CAD build for the part. Positions are in the model's coordinates, mm. A direction names the side the tool comes from. Round coordinates to 2 decimals unless told otherwise and drop trailing zeros. Order: outer loops, then holes, each group sorted by start corner. A loop starts at its lowest first (then second) coordinate and runs counter-clockwise, first axis right, second up. Notation, with made-up numbers: (-3.75, -37.5) -> (24.25, -37.5) arc R31 cw to (24.25, -6.5) -> close; hole circle Ø2 at (82, -5). An arc over 180 degrees is marked (long way). Return JSON: item names as keys, results as strings. Group by question number.
Q1. Cut at B-B (z = -3.75). Write the cut outline in (x, y) (3 decimals), then the cut area to 3 significant figures.
Q2. Cut at C-C (y = 25.4). Write the cut outline in (x, z) (3 decimals).
Q3. Flat gauge pin, fed straight in: pin 1 (4 mm diameter, centred on y = -66.675, z = 3.175, fed in from +X). Where does the tip first touch, or does it go through?
Q4. Cut at A-A (x = 0). Write the cut outline in (y, z) (3 decimals), then the cut area to 3 significant figures.
Q5. Which spindle directions (+Z, -Z, +X, -X, +Y, -Y) get a long thin tool onto all of the face, cutting with end or side? Do faces 5 (the flat face through (-22.225, 1, 0)), 6 (the flat face through (0, 76.2, -10)). Say none if no direction does.
Q6. Mould opens along Y. For faces 1 (the cylindrical face through (-23.835, 28.548, 2.762)), 2 (the flat face through (0, 1, 9.525)), 3 (the flat face through (0, -76.2, -10)), 4 (the cylindrical face through (23.79, 28.548, 2.762)) say: +Y half, -Y half, draft (parallel to the pull), parting line (faces both ways), or undercut.
Q7. Cut at D-D (z = 4.75). Write the cut outline in (x, y) (3 decimals).
Q8. Probe line 1 along X through (y, z) = (-0.5, 3) (3 decimals); line 2 along Z through (x, y) = (5.5, 43.5) (3 decimals). List the from-to ranges inside material, lowest first.
from build123d import *

# Parameters (mm, degrees)
SKETCH1_W           = 50.8
SKETCH1_H           = 25.4
SKETCH1_W_2         = 44.45
SKETCH1_H_2         = 19.05
BOSS_EXTRUDE1_DEPTH = 76.2
SKETCH2_R           = 3.175
CUT_EXTRUDE1_DEPTH  = 93.457395594


with BuildPart() as part:
    # Sketch1 → Boss-Extrude1 (new, symmetric)
    with BuildSketch(Plane(origin=(0, 0, 0), x_dir=(1, 0, 0), z_dir=(0, 1, 0))):
        Rectangle(SKETCH1_W, SKETCH1_H)
        Rectangle(SKETCH1_W_2, SKETCH1_H_2, mode=Mode.SUBTRACT)
    extrude(amount=BOSS_EXTRUDE1_DEPTH, both=True)

    # Sketch2 → Cut-Extrude1 (cut, through all)
    with BuildSketch(Plane.ZY.offset(25.4)):
        with Locations((3.175, -66.675)):
            Circle(SKETCH2_R)
        with Locations((3.175, 25.4)):
            Circle(SKETCH2_R)
    extrude(amount=-CUT_EXTRUDE1_DEPTH, mode=Mode.SUBTRACT)


solid = part.part
Solution:
{
 "1": {"outline": "(-25.4, -76.2) -> (-22.225, -76.2) -> (-22.225, 76.2) -> (-25.4, 76.2) -> close; (22.225, -76.2) -> (25.4, -76.2) -> (25.4, 76.2) -> (22.225, 76.2) -> close", "area": "968 mm²"},
 "2": {"outline": "(-25.4, -12.7) -> (25.4, -12.7) -> (25.4, 0) -> (22.225, 0) -> (22.225, -9.525) -> (-22.225, -9.525) -> (-22.225, 0) -> (-25.4, 0) -> close; (-25.4, 6.35) -> (-22.225, 6.35) -> (-22.225, 9.525) -> (22.225, 9.525) -> (22.225, 6.35) -> (25.4, 6.35) -> (25.4, 12.7) -> (-25.4, 12.7) -> close"},
 "3": {"pin 1": "passes through"},
 "4": {"outline": "(-76.2, -12.7) -> (76.2, -12.7) -> (76.2, -9.525) -> (-76.2, -9.525) -> close; (-76.2, 9.525) -> (76.2, 9.525) -> (76.2, 12.7) -> (-76.2, 12.7) -> close", "area": "968 mm²"},
 "5": {"face 5": "+Y, -Y", "face 6": "+Z, -Z, +X, -X, +Y"},
 "6": {"face 1": "undercut", "face 2": "draft", "face 3": "-Y half", "face 4": "undercut"},
 "7": {"outline": "(-25.4, -76.2) -> (-22.225, -76.2) -> (-22.225, -69.432) -> (-25.4, -69.432) -> close; (-25.4, -63.918) -> (-22.225, -63.918) -> (-22.225, 22.643) -> (-25.4, 22.643) -> close; (-25.4, 28.157) -> (-22.225, 28.157) -> (-22.225, 76.2) -> (-25.4, 76.2) -> close; (22.225, -76.2) -> (25.4, -76.2) -> (25.4, -69.432) -> (22.225, -69.432) -> close; (22.225, -63.918) -> (25.4, -63.918) -> (25.4, 22.643) -> (22.225, 22.643) -> close; (22.225, 28.157) -> (25.4, 28.157) -> (25.4, 76.2) -> (22.225, 76.2) -> close"},
 "8": {"line 1": "x = -25.4 to -22.225, 22.225 to 25.4", "line 2": "z = -12.7 to -9.525, 9.525 to 12.7"}
}
